from build123d import *

# Parameters (mm, degrees)
SKETCH1_R           = 2.38125
SKETCH1_R_2         = 0.75
BOSS_EXTRUDE1_DEPTH = 2


with BuildPart() as part:
    # Sketch1 → Boss-Extrude1 (new, symmetric)
    with BuildSketch(Plane(origin=(0, 0, 0), x_dir=(0, 0, -1), z_dir=(1, 0, 0))):
        with BuildLine():
            Line((-56.625400227, 2.386991318), (-56.625400227, -13.559221537))
            ThreePointArc((-56.625400227, -13.559221537), (-56.966991368, -14.831463057), (-57.899887224, -15.761510537))
            ThreePointArc((-57.899887224, -15.761510537), (-61.589569936, -22.137211246), (-57.899887224, -28.512911956))
            ThreePointArc((-57.899887224, -28.512911956), (-56.966991368, -29.442959435), (-56.625400227, -30.715200956))
            Line((-56.625400227, -30.715200956), (-56.625400227, -43.943749635))
            Line((-56.625400227, -43.943749635), (-43.707520647, -43.943749635))
            Line((-43.707520647, -43.943749635), (-43.707520647, -34.030414011))
            ThreePointArc((-43.707520647, -34.030414011), (-42.567322793, -30.020854914), (-39.487950002, -27.21121463))
            Line((-39.487950002, -27.21121463), (-25.808814493, -20.390042329))
            Line((-25.808814493, -20.390042329), (3.003273, -6.022744555))
            ThreePointArc((3.003273, -6.022744555), (6.576528363, 1.429116992), (0.23290188, 6.72598375))
            Line((0.23290188, 6.72598375), (-43.515144264, 6.72598375))
            ThreePointArc((-43.515144264, 6.72598375), (-46.055144264, 9.26598375), (-43.515144264, 11.80598375))
            Line((-43.515144264, 11.80598375), (-16.803992093, 11.80598375))
            Line((-16.803992093, 11.80598375), (-16.803992093, 18.009025029))
            Line((-16.803992093, 18.009025029), (-52.475776529, 18.009025029))
            ThreePointArc((-52.475776529, 18.009025029), (-51.277962728, 11.814262359), (-54.597011148, 6.44828062))
            ThreePointArc((-54.597011148, 6.44828062), (-56.090099528, 4.65681692), (-56.625400227, 2.386991318))
        make_face()
        Circle(SKETCH1_R, mode=Mode.SUBTRACT)
        with Locations((-45.553086475, -38.863749635)):
            Circle(SKETCH1_R_2, mode=Mode.SUBTRACT)
        with Locations((-47.585086475, -38.863749635)):
            Circle(SKETCH1_R_2, mode=Mode.SUBTRACT)
        with Locations((-49.617086475, -38.863749635)):
            Circle(SKETCH1_R_2, mode=Mode.SUBTRACT)
        with Locations((-51.649086475, -38.863749635)):
            Circle(SKETCH1_R_2, mode=Mode.SUBTRACT)
        with Locations((-54.236184525, -22.137211246)):
            Circle(SKETCH1_R, mode=Mode.SUBTRACT)
        with Locations((-50.410128911, 1.079375692)):
            Circle(SKETCH1_R, mode=Mode.SUBTRACT)
        with Locations((-53.681086475, -38.863749635)):
            Circle(SKETCH1_R_2, mode=Mode.SUBTRACT)
        with BuildLine():
            Line((-36.568397511, 1.976008906), (-19.797694446, -0.914638547))
            Line((-19.797694446, -0.914638547), (-21.730897843, -12.13052726))
            Line((-21.730897843, -12.13052726), (-40.504072916, -8.894727872))
            Line((-40.504072916, -8.894727872), (-38.916021454, 0.318688833))
            ThreePointArc((-38.916021454, 0.318688833), (-38.085451708, 1.633557707), (-36.568397511, 1.976008906))
        make_face(mode=Mode.SUBTRACT)
    extrude(amount=BOSS_EXTRUDE1_DEPTH, both=True)


solid = part.part
Verification items for the finished model (mm, model axes). A direction names the side the tool comes from. Give positions to 0.01 mm unless a question says otherwise; leave off trailing zeros. Order: outer loops, then holes, each group sorted by start corner. A loop starts at its lowest first (then second) coordinate and runs counter-clockwise, first axis right, second up. Notation, with made-up numbers: (56, 10.25) -> (64, 10.25) arc R17 ccw to (64, 25.25) -> close; hole circle Ø2 at (-33, 58). An arc over 180 degrees is marked (long way). Answer as CSV lines item,"result".
Q1. Sectioned sample at C-C on x = 1. Count the separate pieces of the cut face and the enclosed holes in it, plus the area to 3 significant figures.
Solutions:
separate pieces,"1"
enclosed holes,"9"
area,"1,850 mm²"
Q2. Release check for a two-part mould opening along Z. For faces 6 (the cylindrical face through (0.03, 1.31, -6.6)), 7 (the cylindrical face through (0.028, -29.427, 56.976)), 8 (the cylindrical face through (0.028, 1.621, 38.104)) record: +Z half, -Z half, draft (parallel to the pull), parting line (faces both ways), or undercut.
Solutions:
face 6,"-Z half"
face 7,"+Z half"
face 8,"undercut"
Q3. Scan lines: probe 1 along Y at (x, z) = (1.5, 33); probe 2 along Y at (x, z) = (-1.4, 22); probe 3 along Z at (x, y) = (1, -1.5). Record each from-to range of solid material in increasing order.
Solutions:
probe 1,"y = -23.98 to -10.19, 1.36 to 6.73, 11.81 to 18.01"
probe 2,"y = -18.49 to -12.08, -0.54 to 6.73, 11.81 to 18.01"
probe 3,"z = -6.56 to -1.85, 1.85 to 19.9, 39.23 to 56.63"
Q4. Access from +Z, -Z, +X, -X, +Y, -Y to the whole of each face (thin tool, end or side, straight path). Record for faces 1 (the flat face through (-0.03, 0.55, 28.3)), 2 (the flat face through (0, -37, 56.625)), 3 (the flat face through (0, -5, 56.625)), 4 (the flat face through (0, 11.806, 30)), 5 (the flat face through (0, 15, 16.804)).
Solutions:
face 1,"+X, -X"
face 2,"+Z, +X, -X, -Y"
face 3,"+Z, +X, -X, +Y"
face 4,"-Z, +X, -X"
face 5,"-Z, +X, -X, +Y"
Q5. Sectioned sample at D-D on y = -23. Record the cut outline in (x, z).
Solutions:
outline,"(-2, 31.04) -> (2, 31.04) -> (2, 52.02) -> (-2, 52.02) -> close; (-2, 56.46) -> (2, 56.46) -> (2, 61.54) -> (-2, 61.54) -> close"
Q6. Depth check by flat-ended pin: pin 1 (2 mm diameter, centred on x = -0.5, y = -40, fed in from -Z); pin 2 (2 mm diameter, centred on x = 0.5, y = 14, fed in from -Z); pin 3 (1 mm diameter, centred on x = 0.5, z = 3, fed in from -Y). Enter the tip coordinate at first touch or a pass-through.
Solutions:
pin 1,"stops at z = 43.71"
pin 2,"stops at z = 16.8"
pin 3,"stops at y = -9.27"
Q7. Sectioned sample at A-A on y = -10.5. Record the cut outline in (x, z).
Solutions:
outline,"(-2, 5.98) -> (2, 5.98) -> (2, 21.45) -> (-2, 21.45) -> close; (-2, 31.19) -> (2, 31.19) -> (2, 56.63) -> (-2, 56.63) -> close"
Q8. Sectioned sample at B-B on z = 24.5. Record the cut outline in (x, y), plus the area to 3 significant figures.
Solutions:
outline,"(-2, -19.74) -> (2, -19.74) -> (2, -11.65) -> (-2, -11.65) -> close; (-2, -0.1) -> (2, -0.1) -> (2, 6.73) -> (-2, 6.73) -> close; (-2, 11.81) -> (2, 11.81) -> (2, 18.01) -> (-2, 18.01) -> close"
area,"84.5 mm²"
